Part model, mm, in its own coordinate system. A direction names the side the tool comes from. Give positions to 0.01 mm unless a question says otherwise; leave off trailing zeros. Order: outer loops, then holes, each group sorted by start corner. A loop starts at its lowest first (then second) coordinate and runs counter-clockwise, first axis right, second up.
1. Mould opens along Z. For faces 4 (the cylindrical face through (3.94, -9.76, 2.17)), 5 (the cylindrical face through (1.7, 0.1, -2.9)), 6 (the flat face through (16, 4, 4)) say: +Z half, -Z half, draft (parallel to the pull), parting line (faces both ways), or undercut.
2. Slice it at D-D on x = 2. List the corners of the cut face in (y, z).
3. Slice it at A-A on z = 0. List the corners of the cut face in (x, y), and give its area (3 significant figures).
4. Slice it at C-C on x = 15. List the corners of the cut face in (y, z), and give its area (3 significant figures).
5. Drop flat-ended pins along their axis: pin 1 Ø1.7 at (y, z) = (0, 1.5) entering from -X; pin 2 Ø1 at (x, z) = (2.5, 7) entering from +Y; pin 3 Ø1.5 at (x, y) = (6, 4) entering from +Z. Give the stop position or say it passes through.
6. Which spindle directions (+Z, -Z, +X, -X, +Y, -Y) get a long thin tool onto all of the face, cutting with end or side? Do faces 1 (the flat face through (3.5, 0, 0)), 2 (the flat face through (16, 4, -3)), 3 (the cylindrical face through (11.944, -2.749, -5.885)). Say none if no direction does.
7. Probe line 1 (Y direction, x = 1.8, z = 0); line 2 (X direction, y = -4, z = -8); line 3 (X direction, y = 1, z = 1.5). List the from-to ranges inside material, lowest first.
from build123d import *

# Parameters (mm, degrees)
SKETCH_1_R          = 10
EXTRUDE_1_DEPTH     = 8
SKETCH_2_R          = 2.5
EXTRUDE_2_DEPTH     = 8
SKETCH_3_R          = 2.9
CUT_EXTRUDE_1_DEPTH = 3.5


with BuildPart() as part:
    # Эскиз1 → Бобышка-Вытянуть1 (new body)
    with BuildSketch(Plane(origin=(0, 0, 0), x_dir=(0, 0, -1), z_dir=(1, 0, 0))):
        Circle(SKETCH_1_R)
    extrude(amount=EXTRUDE_1_DEPTH)

    # Эскиз2 → Бобышка-Вытянуть2 (add)
    with BuildSketch(Plane(origin=(8, 0, 0), x_dir=(0, 0, -1), z_dir=(1, 0, 0))):
        with Locations((-3.5, 3.5)):
            Circle(SKETCH_2_R)
        with Locations((3.5, 3.5)):
            Circle(SKETCH_2_R)
        with Locations((-3.5, -3.5)):
            Circle(SKETCH_2_R)
        with Locations((3.5, -3.5)):
            Circle(SKETCH_2_R)
    extrude(amount=EXTRUDE_2_DEPTH)

    # Эскиз3 → Вырез-Вытянуть1 (cut)
    with BuildSketch(Plane.ZY):
        Circle(SKETCH_3_R)
    extrude(amount=-CUT_EXTRUDE_1_DEPTH, mode=Mode.SUBTRACT)


solid = part.part
Data:
1. face 4: parting line
1. face 5: undercut
1. face 6: draft
2. outline: circle Ø20 at (0, 0); hole circle Ø5.8 at (0, 0)
3. outline: (0, -10) - (8, -10) - (8, 10) - (0, 10) - (0, 2.9) - (3.5, 2.9) - (3.5, -2.9) - (0, -2.9) - close
3. area: 140 mm2
4. outline: circle Ø5 at (-3.5, -3.5); circle Ø5 at (-3.5, 3.5); circle Ø5 at (3.5, -3.5); circle Ø5 at (3.5, 3.5)
4. area: 78.5 mm2
5. pin 1: stops at x = 3.5
5. pin 2: stops at y = 7.6
5. pin 3: stops at z = 9.46
6. face 1: -X
6. face 2: +Z, -Z, +X, +Y, -Y
6. face 3: +X
7. line 1: y = -10 to -2.9, 2.9 to 10
7. line 2: x = 0 to 8
7. line 3: x = 3.5 to 8
